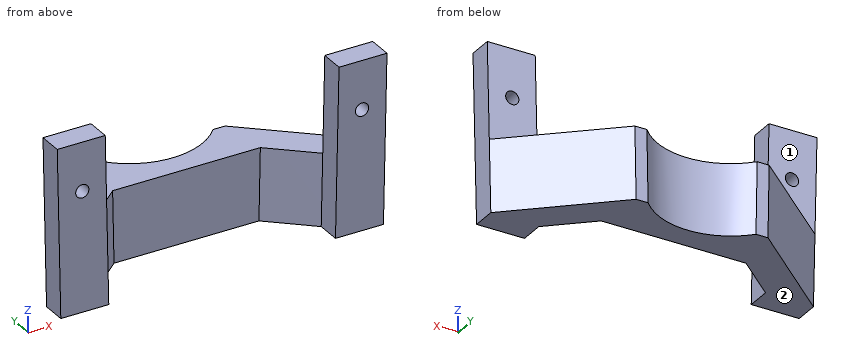
```python
from build123d import *

# Parameters (mm, degrees)
SKETCH1_R             = 2.75
BOSS_EXTRUDE1_DEPTH   = 10
BOSS_EXTRUDE1_2_DEPTH = 10


with BuildPart() as part:
    # Sketch1 → Boss-Extrude1 (new body)
    with BuildSketch(Plane(origin=(0, 0, 0), x_dir=(1, 0, 0), z_dir=(0, 1, 0))):
        Polygon((0, 0), (20.004497681, 0), (21.489122754, 70), (1.484625073, 70), align=None)
        with Locations((10.430924608, 20.212041611)):
            Circle(SKETCH1_R, mode=Mode.SUBTRACT)
    extrude(amount=BOSS_EXTRUDE1_DEPTH)



with BuildPart() as body_2:
    # Sketch1 → Boss-Extrude1 2 (new body)
    with BuildSketch(Plane(origin=(0, 0, 0), x_dir=(1, 0, 0), z_dir=(0, 1, 0))):
        Polygon((116.0383729, 70), (136.042870581, 70), (137.527495654, 0), (117.522997972, 0), align=None)
        with Locations((127.096571045, 20.212041611)):
            Circle(SKETCH1_R, mode=Mode.SUBTRACT)
    extrude(amount=BOSS_EXTRUDE1_2_DEPTH)


with BuildPart() as part_1:
    add(part.part)

    add(body_2.part)  # Loft1 merges body 2
    # Sketch2 → Loft1 section 0
    with BuildSketch(Plane(origin=(0, 0, -70), x_dir=(-1, 0, 0), z_dir=(0, 0, -1))):
        with BuildLine():
            Line((-91.263747827, 45), (-96.263747827, 45))
            Line((-96.263747827, 45), (-136.042870581, 10))
            Line((-136.042870581, 10), (-116.0383729, 10))
            Line((-116.0383729, 10), (-98.990177434, 25))
            Line((-98.990177434, 25), (-38.53731822, 25))
            Line((-38.53731822, 25), (-21.489122754, 10))
            Line((-21.489122754, 10), (-1.484625073, 10))
            Line((-1.484625073, 10), (-41.263747827, 45))
            Line((-41.263747827, 45), (-46.263747827, 45))
            ThreePointArc((-46.263747827, 45), (-68.763747827, 35), (-91.263747827, 45))
        make_face()
    # Sketch3 → Loft1 section 1
    with BuildSketch(Plane(origin=(0, 0, -40), x_dir=(-1, 0, 0), z_dir=(0, 0, -1))):
        with BuildLine():
            Line((-136.679138469, 10), (-96.763747827, 45))
            Line((-96.763747827, 45), (-91.763747827, 45))
            ThreePointArc((-91.763747827, 45), (-68.763747827, 34.627036727), (-45.763747827, 45))
            Line((-45.763747827, 45), (-40.763747827, 45))
            Line((-40.763747827, 45), (-0.848357184, 10))
            Line((-0.848357184, 10), (-20.852854866, 10))
            Line((-20.852854866, 10), (-37.959450855, 25))
            Line((-37.959450855, 25), (-99.568044798, 25))
            Line((-99.568044798, 25), (-116.674640788, 10))
            Line((-116.674640788, 10), (-136.679138469, 10))
        make_face()
    loft()


solid = part_1.part
```
Verification items for the finished model (mm, model axes). Face numbers are marked on the shaded views. A direction names the side the tool comes from. Give positions to 0.01 mm unless a question says otherwise; leave off trailing zeros. Order: outer loops, then holes, each group sorted by start corner. A loop starts at its lowest first (then second) coordinate and runs counter-clockwise, first axis right, second up. Notation, with made-up numbers: (72.5, 23.25) - (103.5, 23.25) arc R20 ccw to (103.5, 60.25) - close; hole circle Ø6 at (-28.5, -8.75). An arc over 180 degrees is marked (long way). Answer as CSV lines item,"result". Start each with the question number.
Item 1: Section check A-A, the plane z = -6.5. Record the boundary of the cut face in (x, y), plus the area to 3 significant figures.
Item 2: Gauge pin test, flat ends, axial feed: pin 1 (6.5 mm diameter, centred on x = 131.5, z = -22.5, fed in from +Y); pin 2 (1.5 mm diameter, centred on x = 88.5, z = -60, fed in from +Y); pin 3 (5 mm diameter, centred on y = 21, z = -52, fed in from +X); pin 4 (5 mm diameter, centred on x = 10.43, z = -20.21, fed in from -Y). Record the tip position at first contact, or that the pin passes through.
Item 3: Access from +Z, -Z, +X, -X, +Y, -Y to the whole of each face (thin tool, end or side, straight path). Record for the marked faces 1 and 2.
Item 4: Material ranges on L1, parallel to X at y = 2, z = -22; L2, parallel to X at y = 15.5, z = -54; L3, parallel to Z at x = 96, y = 43, recorded low to high.
Filled in:
1,outline,"(0.14, 0) - (20.14, 0) - (20.14, 10) - (0.14, 10) - close; (117.39, 0) - (137.39, 0) - (137.39, 10) - (117.39, 10) - close"
1,area,"400 mm^2"
2,pin 1,"y = 10"
2,pin 2,"y = 42.8"
2,pin 3,"x = 126.74"
2,pin 4,"through"
3,face 1,"+Z, +X, -X, +Y"
3,face 2,"-Z, +X, -X, +Y, -Y"
4,L1,"0.47 to 8.34, 12.52 to 20.47, 117.06 to 125.01, 129.19 to 137.06"
4,L2,"7.41 to 27.41, 110.12 to 130.12"
4,L3,"-70 to -40"
